Can you work these out from the model? Positions are in its coordinate system, mm. A direction names the side the tool comes from. Coordinates: 2 decimals unless noted, no trailing zeros. Write each loop counter-clockwise with the first axis right and the second up, starting at its lowest first coordinate (ties: lowest second). Pieces come first, ordered by that corner, then holes. Notation, with made-up numbers: (-31.75, 75.5) - (20.25, 75.5) arc R19 cw to (20.25, 97.5) - close; hole circle Ø10 at (40.25, 28). An arc over 180 degrees is marked (long way). Write each question's results on one line, items separated by ' | '. Start each with the question number.
Autodesk Inventor part; units mm, degrees
ref_plane "РабПлоскость1" through (36.5, 0, 0) normal (1, 0, 0) x (0, 0, -1)
ref_plane "YZ Plane" through (0, 0, 0) normal (1, 0, 0) x (0, 1, 0)
ref_plane "XZ Plane" through (0, 0, 0) normal (0, 1, 0) x (-1, 0, 0)
sketch "Эскиз1" plane through (0, 0, 0) normal (1, 0, 0) x (0, 1, 0)
  circle A0 centre (0, 0) radius 27
  dimension "d0" = 54
extrude "Выдавливание1" add sketch "Эскиз1" along normal blind 16.5
ref_plane "РабПлоскость1" through (36.5, 0, 0) normal (1, 0, 0) x (0, 0, -1)
sketch "Эскиз2" plane through (36.5, 0, 0) normal (1, 0, 0) x (0, 0, -1)
  circle A0 centre (0, 47.75) radius 33.9
  point P0 (0, 0)
  dimension "d4" = 67.8
  dimension "d5" = 47.75
extrude "Выдавливание2" add sketch "Эскиз2" along normal blind 15.5
sketch "Эскиз3" plane through (36.5, 47.75, 0) normal (-1, 0, 0) x (0, 0, 1)
  circle A0 centre (0, 0) radius 33.9
  arc A1 (-29.6851, -52.0851) -> (29.6851, -52.0851) centre (0, -47.75) ccw
  circle A2 centre (0, -47.75) radius 27
  line L0 (36.5127, -5.3321) -> (29.6851, -52.0851)
  line L1 (-36.5127, -5.3321) -> (-29.6851, -52.0851)
  arc A3 (36.5127, -5.3321) -> (-36.5127, -5.3321) centre (0, 0) ccw
  dimension "d11" = 3
  dimension "d12" = 3
extrude "Выдавливание3" add sketch "Эскиз3" along normal up to surface (20 mm away) contours A0 A2 | A2 A0 | A0 A2 | L1 A3 L0 A1
sketch "Эскиз15" plane through (36.5, 47.75, 0) normal (1, 0, 0) x (0, 0, -1)
  arc A0 (0, 94) -> (-83.379, 43.4044) centre (0, 0) ccw
  line L0 (-83.379, 43.4044) -> (0, 0)
  line L1 (0, -114.4319) -> (0, 142.3414)
  arc A1 (83.379, 43.4044) -> (0, 94) centre (0, 0) ccw
  line L2 (83.379, 43.4044) -> (0, 0)
  arc A2 (36.5127, -5.3321) -> (-36.5127, -5.3321) centre (0, 0) ccw
  arc A3 (32.7307, 17.0385) -> (-32.7307, 17.0385) centre (0, 0) ccw
  point P0 (0, -47.75)
  dimension "d66" = 94
  dimension "d67" = 62.5
extrude "Выдавливание10" add sketch "Эскиз15" against normal up to surface (20 mm away) contours L1 A2 L0 A0 | A1 L2 A2 L1
sketch "Эскиз4" plane through (0, 0, 0) normal (0, 0, 1) x (1, 0, 0)
  line L0 (16.5, 31.9847) -> (31.5, 78.15)
  line L1 (31.5, 78.15) -> (31.5, 84.65)
  line L2 (36.5, 84.65) -> (16.5, 84.65)
  line L3 (31.5, 84.65) -> (31.0691, 84.65)
  line L4 (36.5, 84.65) -> (36.5, 42.4179)
  line L5 (16.5, 84.65) -> (16.5, 42.4179)
  line L6 (16.5, 84.65) -> (16.5, 31.9847)
  line L7 (36.5, -30) -> (16.5, -30)
  line L8 (21.5, -30) -> (21.5, -21)
  line L9 (21.5, -21) -> (36.5, 4.9808)
  line L10 (36.5, 4.9808) -> (36.5, -30)
  line L11 (36.5, -30) -> (21.5, -30)
  line L12 (16.5, -4.3351) -> (16.5, -30)
  point P0 (0, 0)
  dimension "d23" = 5
  dimension "d24" = 6.5
  dimension "d25" = 72
  dimension "d26" = 60
  dimension "d27" = 5
  dimension "d28" = 9
extrude "Выдавливание5" cut sketch "Эскиз4" along normal through all both and the other way through all contours L7 L8 L9 L10
mirror "Зеркальное отражение5" about plane through (0, 0, 0) normal (-1, 0, 0) of "Выдавливание3", "Выдавливание2", "Выдавливание10", "Выдавливание5", "Выдавливание1"
move or copy body "Переместить тело3" bodies to move or copy 1 copy no translate (0, -47.75, 0)
properties part number "crankshaft" material "Сталь, высокопрочная, низколегированная"
Q1. I need wall thicknesses on line 1 along X through (y, z) = (46, -48.5); line 2 along X through (y, z) = (-5.5, 31); line 3 along Z through (x, y) = (-35, -42). Which ranges of each line are inside material? Lowest first, please. Write a range as from..to.
Q2. For faces 1 (the face through (52, 0, 0)), 2 (the face through (21.5, -72, 0)), which set-ups out of +Z, -Z, +X, -X, +Y, -Y let a thin tool reach every point of the face, with its end or its side?
Q3. If we section it at A-A (y = 0): Please give me the cut outline in (x, z), then the cut area to 3 significant figures.
Q4. If we section it at D-D (x = 43): Please give me the cut outline in (y, z), then the cut area to 3 significant figures.
Q5. If we section it at C-C (y = -47.75): Please give me the cut outline in (x, z).
Q6. I'm going to push flat-ended pins straight in: pin 1 Ø10 at (x, y) = (22.5, 28) entering from -Z; pin 2 Ø10 at (y, z) = (-73, 1.5) entering from +X; pin 3 Ø2 at (x, z) = (14, -18) entering from +Y. Where does each tip first touch, or does it pass through?
Q7. If we section it at B-B (z = -71): Please give me the cut outline in (x, y), then the cut area to 3 significant figures.
Q8. Thinking about a two-plate mould opening in Y: for faces 3 (the face through (26.64, 5.99, -36.41)), 4 (the face through (-44.142, 22.911, 24.986)), 5 (the face through (28.895, -55.941, -0.435)), 6 (the face through (-21.5, -72, 0)), which applies, pulls with the +Y half, pulls with the -Y half, needs draft (parallel to the pull), parting line crosses it, or undercut?
Answer list:
1) line 1: x = -36.5..-16.5, 16.5..36.5 | line 2: x = -52..-16.5, 16.5..52 | line 3: z = -31.16..31.16
2) face 1: +Z, -Z, +X, +Y, -Y | face 2: +Z, -Z, +X, -Y
3) outline: (-52, -33.9) - (-36.5, -33.9) - (-36.5, -36.9) - (-16.5, -36.9) - (-16.5, 36.9) - (-36.5, 36.9) - (-36.5, 33.9) - (-52, 33.9) - close; (16.5, -36.9) - (36.5, -36.9) - (36.5, -33.9) - (52, -33.9) - (52, 33.9) - (36.5, 33.9) - (36.5, 36.9) - (16.5, 36.9) - close | area: 5,050 mm2
4) outline: circle Ø67.8 at (0, 0) | area: 3,610 mm2
5) outline: (-33.62, -30.32) - (-16.5, -30.32) - (-16.5, -27) - (16.5, -27) - (16.5, -30.32) - (33.62, -30.32) - (33.62, 30.32) - (16.5, 30.32) - (16.5, 27) - (-16.5, 27) - (-16.5, 30.32) - (-33.62, 30.32) - close
6) pin 1: stops at z = -63.39 | pin 2: stops at x = 21.93 | pin 3: stops at y = -26.77
7) outline: (-36.5, 36.96) - (-16.5, 36.96) - (-16.5, 61.6) - (-36.5, 61.6) - close; (16.5, 36.96) - (36.5, 36.96) - (36.5, 61.6) - (16.5, 61.6) - close | area: 986 mm2
8) face 3: undercut | face 4: parting line crosses it | face 5: pulls with the -Y half | face 6: needs draft
